from build123d import *

# Parameters (mm, degrees)
BOSS_EXTRUDE1_DEPTH        = 15
F_20_0MM_DOWEL_HOLE2_D     = 20
F_20_0MM_DOWEL_HOLE2_DEPTH = 22.25
F_20_0MM_DOWEL_HOLE2_TIP   = 6.00860619
F_20_0MM_DOWEL_HOLE1_D     = 20
F_20_0MM_DOWEL_HOLE1_DEPTH = 22.25
F_20_0MM_DOWEL_HOLE1_TIP   = 6.00860619


with BuildPart() as part:
    # Sketch1 → Boss-Extrude1 (new body)
    with BuildSketch(Plane.XY):
        Polygon((0, 0), (-220, 0), (-220, -35), (-35, -35), (-35, -270), (0, -270), align=None)
    extrude(amount=BOSS_EXTRUDE1_DEPTH)

    # Ø20.0mm Dowel Hole2
    with Locations(Plane.XY.offset(15)):
        with Locations((-17.5, -17.5), (-202.5, -17.5), (-17.5, -252.5)):
            Hole(F_20_0MM_DOWEL_HOLE2_D / 2, depth=F_20_0MM_DOWEL_HOLE2_DEPTH)
            with Locations((0, 0, -(F_20_0MM_DOWEL_HOLE2_DEPTH + F_20_0MM_DOWEL_HOLE2_TIP / 2))):  # 118° drill point
                Cone(0, F_20_0MM_DOWEL_HOLE2_D / 2, F_20_0MM_DOWEL_HOLE2_TIP, mode=Mode.SUBTRACT)

    # Ø20.0mm Dowel Hole1
    with Locations(Plane.XY.offset(15)):
        with Locations((-17.5, -17.5), (-202.5, -17.5), (-17.5, -252.5)):
            Hole(F_20_0MM_DOWEL_HOLE1_D / 2, depth=F_20_0MM_DOWEL_HOLE1_DEPTH)
            with Locations((0, 0, -(F_20_0MM_DOWEL_HOLE1_DEPTH + F_20_0MM_DOWEL_HOLE1_TIP / 2))):  # 118° drill point
                Cone(0, F_20_0MM_DOWEL_HOLE1_D / 2, F_20_0MM_DOWEL_HOLE1_TIP, mode=Mode.SUBTRACT)


solid = part.part
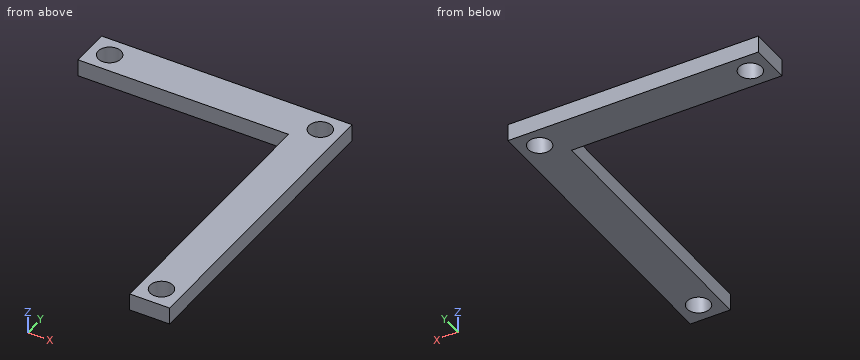
Work out the finished part from the listing and answer in its coordinate system (mm). Give positions to 0.01 mm unless a question says otherwise; leave off trailing zeros. Loops run counter-clockwise (first coordinate to the right, second up) from the corner with the lowest first, then second, coordinate; pieces in that order, holes last. Notation, with made-up numbers: (66.25, 89.25) -> (88.25, 89.25) arc R24 cw to (88.25, 110.25) -> close; hole circle Ø1 at (13.5, 84). An arc over 180 degrees is marked (long way). Use a Markdown table: item, result. Add a question column.
1) Each of these flat-tipped pins is pushed along its axis until it touches: P1, Ø4.5, axis at x = -94, z = 4, coming from the -Y side; P2, Ø6, axis at y = -92, z = 9, coming from the -X side. Where does it stop, or does it pass through?
2) Consider line 1 along Y through (x, z) = (-17.5, 9.5); line 2 along X through (y, z) = (-129.5, 2.75). Determine where each line is inside the solid, lowest interval first.
3) The part is cut by section B-B, the plane y = -17.5. Determine the outline of the cut face in (x, z).
4) The part is cut by section D-D, the plane z = 8.25. Determine the outline of the cut face in (x, y).
5) The part is cut by section A-A, the plane y = -252.5. Determine the outline of the cut face in (x, z).
Reported:
| question | item | result |
|---|---|---|
| 1 | P1 | stops at y = -35 |
| 1 | P2 | stops at x = -35 |
| 2 | line 1 | y = -270 to -262.5, -242.5 to -27.5, -7.5 to 0 |
| 2 | line 2 | x = -35 to 0 |
| 3 | outline | (-220, 0) -> (-212.5, 0) -> (-212.5, 15) -> (-220, 15) -> close; (-192.5, 0) -> (-27.5, 0) -> (-27.5, 15) -> (-192.5, 15) -> close; (-7.5, 0) -> (0, 0) -> (0, 15) -> (-7.5, 15) -> close |
| 4 | outline | (-220, -35) -> (-35, -35) -> (-35, -270) -> (0, -270) -> (0, 0) -> (-220, 0) -> close; hole circle Ø20 at (-202.5, -17.5); hole circle Ø20 at (-17.5, -252.5); hole circle Ø20 at (-17.5, -17.5) |
| 5 | outline | (-35, 0) -> (-27.5, 0) -> (-27.5, 15) -> (-35, 15) -> close; (-7.5, 0) -> (0, 0) -> (0, 15) -> (-7.5, 15) -> close |
